Geometry check sheet. Reference: the model listing, model coordinates, mm. A direction names the side the tool comes from. Round coordinates to 2 decimals unless told otherwise and drop trailing zeros. Write each loop counter-clockwise with the first axis right and the second up, starting at its lowest first coordinate (ties: lowest second). Pieces come first, ordered by that corner, then holes.
Item 1: Draft check along X on faces 6 (the face through (262, 1.3, -12)), 7 (the face through (0, 4, -4)), 8 (the face through (79, 3.3, -12)). Enter one of: pulls with the +X half, pulls with the -X half, needs draft (parallel to the pull), parting line crosses it, or undercut.
Item 2: Cross-section at A-A (x = 118.5). Enter the section's corners in (y, z).
Item 3: Depth check by flat-ended pin: P1, Ø6, axis at y = 6.3, z = -12.4, coming from the +X side; P2, Ø2, axis at y = 2.5, z = -14, coming from the -X side; P3, Ø2.5, axis at x = 327, y = 12.5, coming from the +Z side; P4, Ø8, axis at y = 10.5, z = -10, coming from the +X side. Enter the tip coordinate at first touch or a pass-through.
Item 4: Access from +Z, -Z, +X, -X, +Y, -Y to the whole of each face (thin tool, end or side, straight path). Record for faces 1 (the face through (140, 12, -1.3)), 2 (the face through (168, 4, 0)), 3 (the face through (168, 0, -4)), 4 (the face through (201, 3.3, -12)), 5 (the face through (79, 1.3, -12)).
Item 5: Scan lines: probe 1 along X at (y, z) = (13.5, -9.25); probe 2 along Y at (x, z) = (325.75, -2.5); probe 3 along Z at (x, y) = (136.75, 2.85). Record each from-to range of solid material in increasing order.
from build123d import *

# Parameters (mm, degrees)
SKETCH1_W           = 8.5
SKETCH1_H           = 8.5
BOSS_EXTRUDE1_DEPTH = 340.5
SKETCH2_W           = 15
SKETCH2_H           = 2
BOSS_EXTRUDE2_DEPTH = 7.8
SKETCH3_R           = 1.95
CUT_EXTRUDE1_DEPTH  = 7.8
SKETCH4_W           = 15
SKETCH4_H           = 2
BOSS_EXTRUDE3_DEPTH = 7.8
SKETCH5_R           = 1.95
CUT_EXTRUDE2_DEPTH  = 7.8
FILLET1_R           = 1
FILLET3_R           = 1
BOSS_EXTRUDE5_DEPTH = 2.2
BOSS_EXTRUDE6_DEPTH = 2.2
SKETCH9_R           = 1.95
CUT_EXTRUDE3_DEPTH  = 350


with BuildPart() as part:
    # Sketch1 → Boss-Extrude1 (new body)
    with BuildSketch(Plane(origin=(0, 0, 0), x_dir=(0, 0, -1), z_dir=(1, 0, 0))):
        with Locations((4.25, 4.25)):
            Rectangle(SKETCH1_W, SKETCH1_H)
    extrude(amount=BOSS_EXTRUDE1_DEPTH)

    # Sketch2 → Boss-Extrude2 (add)
    with BuildSketch(Plane(origin=(0, 8.5, 0), x_dir=(1, 0, 0), z_dir=(0, 1, 0))):
        with Locations((17.75, 2.3)):
            Rectangle(SKETCH2_W, SKETCH2_H)
        with Locations((78.75, 2.3)):
            Rectangle(SKETCH2_W, SKETCH2_H)
        with Locations((139.75, 2.3)):
            Rectangle(SKETCH2_W, SKETCH2_H)
        with Locations((200.75, 2.3)):
            Rectangle(SKETCH2_W, SKETCH2_H)
        with Locations((261.75, 2.3)):
            Rectangle(SKETCH2_W, SKETCH2_H)
        with Locations((322.75, 2.3)):
            Rectangle(SKETCH2_W, SKETCH2_H)
    extrude(amount=BOSS_EXTRUDE2_DEPTH)

    # Sketch3 → Cut-Extrude1 (cut)
    with BuildSketch(Plane.XY.offset(-1.3)):
        with Locations((14.75, 12.4)):
            Circle(SKETCH3_R)
        with Locations((20.75, 12.4)):
            Circle(SKETCH3_R)
        with Locations((75.75, 12.4)):
            Circle(SKETCH3_R)
        with Locations((81.75, 12.4)):
            Circle(SKETCH3_R)
        with Locations((136.75, 12.4)):
            Circle(SKETCH3_R)
        with Locations((142.75, 12.4)):
            Circle(SKETCH3_R)
        with Locations((197.75, 12.4)):
            Circle(SKETCH3_R)
        with Locations((203.75, 12.4)):
            Circle(SKETCH3_R)
        with Locations((258.75, 12.4)):
            Circle(SKETCH3_R)
        with Locations((264.75, 12.4)):
            Circle(SKETCH3_R)
        with Locations((319.75, 12.4)):
            Circle(SKETCH3_R)
        with Locations((325.75, 12.4)):
            Circle(SKETCH3_R)
    extrude(amount=-CUT_EXTRUDE1_DEPTH, mode=Mode.SUBTRACT)

    # Sketch4 → Boss-Extrude3 (add)
    with BuildSketch(Plane(origin=(0, 0, -8.5), x_dir=(-1, 0, 0), z_dir=(0, 0, -1))):
        with Locations((-261.75, 2.3)):
            Rectangle(SKETCH4_W, SKETCH4_H)
        with Locations((-322.75, 2.3)):
            Rectangle(SKETCH4_W, SKETCH4_H)
        with Locations((-200.75, 2.3)):
            Rectangle(SKETCH4_W, SKETCH4_H)
        with Locations((-139.75, 2.3)):
            Rectangle(SKETCH4_W, SKETCH4_H)
        with Locations((-78.75, 2.3)):
            Rectangle(SKETCH4_W, SKETCH4_H)
        with Locations((-17.75, 2.3)):
            Rectangle(SKETCH4_W, SKETCH4_H)
    extrude(amount=BOSS_EXTRUDE3_DEPTH)

    # Sketch5 → Cut-Extrude2 (cut)
    with BuildSketch(Plane.XZ.offset(-1.3)):
        with Locations(Location((264.75, -12.4, 0), (0, 0, 270))):
            Circle(SKETCH5_R)
        with Locations(Location((258.75, -12.4, 0), (0, 0, 270))):
            Circle(SKETCH5_R)
        with Locations(Location((203.75, -12.4, 0), (0, 0, 270))):
            Circle(SKETCH5_R)
        with Locations(Location((197.75, -12.4, 0), (0, 0, 270))):
            Circle(SKETCH5_R)
        with Locations(Location((142.75, -12.4, 0), (0, 0, 270))):
            Circle(SKETCH5_R)
        with Locations(Location((136.75, -12.4, 0), (0, 0, 270))):
            Circle(SKETCH5_R)
        with Locations(Location((20.75, -12.4, 0), (0, 0, 270))):
            Circle(SKETCH5_R)
        with Locations(Location((14.75, -12.4, 0), (0, 0, 270))):
            Circle(SKETCH5_R)
        with Locations(Location((81.75, -12.4, 0), (0, 0, 270))):
            Circle(SKETCH5_R)
        with Locations(Location((75.75, -12.4, 0), (0, 0, 270))):
            Circle(SKETCH5_R)
        with Locations(Location((325.75, -12.4, 0), (0, 0, 270))):
            Circle(SKETCH5_R)
        with Locations(Location((319.75, -12.4, 0), (0, 0, 270))):
            Circle(SKETCH5_R)
    extrude(amount=-CUT_EXTRUDE2_DEPTH, mode=Mode.SUBTRACT)

    # Fillet1
    fillet1_edges = [part.edges().sort_by_distance(p)[0] for p in [
        (340.5, 4.25, -8.5),
        (340.5, 8.5, -4.25),
        (340.5, 4.25, 0),
        (340.5, 0, -4.25),
    ]]
    fillet(fillet1_edges, radius=FILLET1_R)

    # Fillet3
    fillet3_edges = [part.edges().sort_by_distance(p)[0] for p in [
        (0, 8.5, -4.25),
        (0, 4.25, -8.5),
        (0, 0, -4.25),
        (0, 4.25, 0),
    ]]
    fillet(fillet3_edges, radius=FILLET3_R)

    # Sketch7 → Boss-Extrude5 (add)
    with BuildSketch(Plane(origin=(330.25, 0, 0), x_dir=(0, 0, -1), z_dir=(1, 0, 0))):
        Polygon((1.3, 8.5), (8.5, 8.5), (8.5, 1.3), (16.3, 1.3), (16.3, 16.3), (1.3, 16.3), align=None)
    extrude(amount=BOSS_EXTRUDE5_DEPTH)

    # Sketch8 → Boss-Extrude6 (add)
    with BuildSketch(Plane.ZY.offset(-10.25)):
        Polygon((-1.3, 16.3), (-16.3, 16.3), (-16.3, 1.3), (-8.5, 1.3), (-8.5, 8.5), (-1.3, 8.5), align=None)
    extrude(amount=BOSS_EXTRUDE6_DEPTH)

    # Sketch9 → Cut-Extrude3 (cut)
    with BuildSketch(Plane.ZY.offset(-8.05)):
        with Locations((-12.4, 6.3)):
            Circle(SKETCH9_R)
        with Locations((-6.3, 12.4)):
            Circle(SKETCH9_R)
    extrude(amount=-CUT_EXTRUDE3_DEPTH, mode=Mode.SUBTRACT)


solid = part.part
Resolved:
1. face 6: needs draft
1. face 7: pulls with the -X half
1. face 8: undercut
2. outline: (0, -8.5) - (8.5, -8.5) - (8.5, 0) - (0, 0) - close
3. P1: stops at x = 332.45
3. P2: stops at x = 8.05
3. P3: stops at z = -1.3
3. P4: stops at x = 340.5
4. face 1: +Z, +X, -X, +Y
4. face 2: +Z, +X, -X, +Y, -Y
4. face 3: +Z, -Z, +X, -X, -Y
4. face 4: -Z, +Y
4. face 5: -Z, +X, -X, -Y
5. probe 1: x = 8.05 to 10.25, 330.25 to 332.45
5. probe 2: y = 0 to 10.45, 14.35 to 16.3
5. probe 3: z = -16.3 to -14.35, -10.45 to 0
